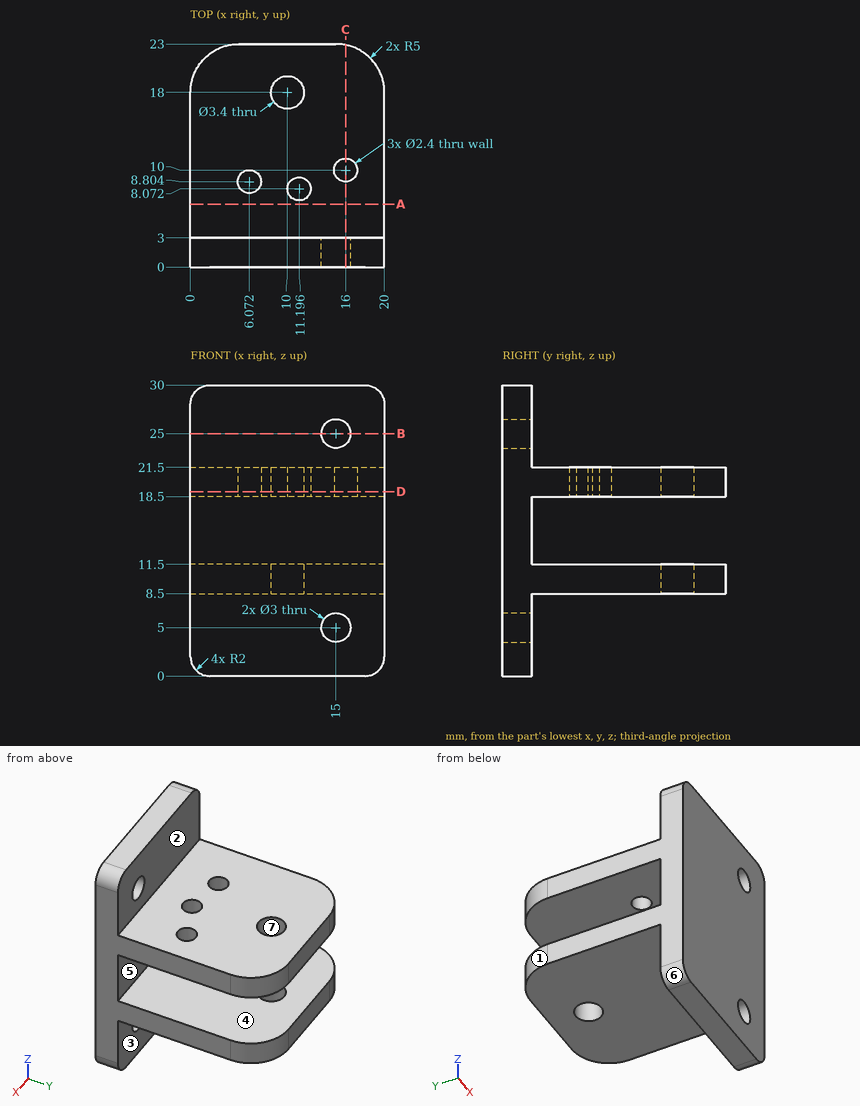
Design review of the part shown in the three views and the two pictorial views. Dimensions are in mm from the part's minimum x, y and z. A direction names the side the tool comes from. Give positions to 0.01 mm unless a question says otherwise; leave off trailing zeros. Loops run counter-clockwise (first coordinate to the right, second up) from the corner with the lowest first, then second, coordinate; pieces in that order, holes last. Notation, with made-up numbers: M 73,50.25 L 104,50.25 A19 ccw 104,57.25 Z; hole C -25.75,37 d4. An arc over 180 degrees is marked long. Answer as a JSON object with one key per item and string values.
Item 1: We need section B-B (z = 25). State the section outline as (x, y) points.
Output values:
{"outline": "M 0,0 L 13.5,0 L 13.5,3 L 0,3 Z; M 16.5,0 L 20,0 L 20,3 L 16.5,3 Z"}
Item 2: We need section D-D (z = 19). State the section outline as (x, y) points, and give its area (3 significant figures).
Output values:
{"outline": "M 0,0 L 20,0 L 20,18 A5 ccw 15,23 L 5,23 A5 ccw 0,18 Z; hole C 6.07,8.8 d2.4; hole C 10,18 d3.4; hole C 11.2,8.07 d2.4; hole C 16,10 d2.4", "area": "427 mm2"}
Item 3: For P1, Ø1.4, axis at x = 11.2, y = 8.07, coming from the +Z side; P2, Ø4, axis at x = 6.5, z = 25, coming from the +Y side; P3, Ø1.9, axis at x = 6.07, y = 8.8, coming from the -Z side, all flat-tipped, find the tip position at first contact; note any pin that passes through.
Output values:
{"P1": "stops at z = 11.5", "P2": "stops at y = 3", "P3": "stops at z = 8.5"}
Item 4: Machinability: for the marked faces 1, 2, 3 and 4, which of the approach directions +Z, -Z, +X, -X, +Y, -Y give a long, thin tool a straight path to every point of the face, cutting with its end or side? Answer none if there is none.
Output values:
{"face 1": "+Z, -Z, -X, +Y", "face 2": "+Z, +X, -X, +Y", "face 3": "-Z, +X, -X, +Y", "face 4": "+X, -X, +Y"}
Item 5: Mouldability with a two-part tool opening along X and no side actions: class the marked faces 5, 6 and 7 as pulls with the +X half, pulls with the -X half, needs draft (parallel to the pull), parting line crosses it, or undercut.
Output values:
{"face 5": "needs draft", "face 6": "pulls with the -X half", "face 7": "undercut"}
Item 6: Wall thickness on line 1 along X through (y, z) = (18, 9.95); line 2 along Z through (x, y) = (18.5, 4); line 3 along Y through (x, z) = (18.5, 16.5): over which ranges is each line inside the solid? List them lowest first.
Output values:
{"line 1": "x = 0 to 8.3, 11.7 to 20", "line 2": "z = 8.5 to 11.5, 18.5 to 21.5", "line 3": "y = 0 to 3"}
Item 7: We need section A-A (y = 6.5). State the section outline as (x, z) points, and give its area (3 significant figures).
Output values:
{"outline": "M 0,8.5 L 20,8.5 L 20,11.5 L 0,11.5 Z; M 0,18.5 L 20,18.5 L 20,21.5 L 0,21.5 Z", "area": "120 mm2"}
Item 8: We need section C-C (x = 16). State the section outline as (y, z) points.
Output values:
{"outline": "M 0,0 L 3,0 L 3,3.88 L 0,3.88 Z; M 0,6.12 L 3,6.12 L 3,8.5 L 22.9,8.5 L 22.9,11.5 L 3,11.5 L 3,18.5 L 8.8,18.5 L 8.8,21.5 L 3,21.5 L 3,23.88 L 0,23.88 Z; M 0,26.12 L 3,26.12 L 3,30 L 0,30 Z; M 11.2,18.5 L 22.9,18.5 L 22.9,21.5 L 11.2,21.5 Z"}
